```python
from build123d import *

# Parameters (mm, degrees)
BOSS_EXTRUDE1_DEPTH = 6.35
SKETCH3_R           = 2.75
CUT_EXTRUDE1_DEPTH  = 7.35


with BuildPart() as part:
    # Sketch2 → Boss-Extrude1 (new body)
    with BuildSketch(Plane(origin=(0, 0, 0), x_dir=(0, 0, -1), z_dir=(1, 0, 0))):
        Polygon((34.047619048, 160), (95.952380952, 160), (130, 50), (130, 0), (0, 0), (0, 50), align=None)
    extrude(amount=BOSS_EXTRUDE1_DEPTH)

    # Sketch3 → Cut-Extrude1 (cut, through all)
    with BuildSketch(Plane(origin=(6.35, 0, 0), x_dir=(0, 0, -1), z_dir=(1, 0, 0))):
        with Locations((10, 42.5)):
            Circle(SKETCH3_R)
        with Locations((45, 42.5)):
            Circle(SKETCH3_R)
        with Locations((10, 7.5)):
            Circle(SKETCH3_R)
        with Locations((45, 7.5)):
            Circle(SKETCH3_R)
        with Locations((120, 7.5)):
            Circle(SKETCH3_R)
        with Locations((85, 7.5)):
            Circle(SKETCH3_R)
        with Locations((85, 42.5)):
            Circle(SKETCH3_R)
        with Locations((120, 42.5)):
            Circle(SKETCH3_R)
    extrude(amount=-CUT_EXTRUDE1_DEPTH, mode=Mode.SUBTRACT)


solid = part.part
```
Model file for the job. Use its own axes, mm. Round coordinates to 2 decimals unless told otherwise and drop trailing zeros. Write each loop counter-clockwise with the first axis right and the second up, starting at its lowest first coordinate (ties: lowest second). Pieces come first, ordered by that corner, then holes. Notation, with made-up numbers: (31, 25.5) -> (40, 25.5) arc R14 cw to (40, 38.5) -> close; hole circle Ø11 at (42, 32). An arc over 180 degrees is marked (long way). Answer as CSV lines item,"result".
1. Drill centre lines: line 1 (Y direction, x = 4.5, z = -45); line 2 (Z direction, x = 1.5, y = 9); line 3 (Z direction, x = 5, y = 103). Where is each one in solid material? Low to high.
Resolved:
line 1,"0 to 4.75, 10.25 to 39.75, 45.25 to 160"
line 2,"-130 to -122.3, -117.7 to -87.3, -82.7 to -47.3, -42.7 to -12.3, -7.7 to 0"
line 3,"-113.6 to -16.4"
2. Slice it at B-B, the plane x = 3.25. State how many separate pieces and enclosed holes the cut face has, plus the area to 3 significant figures.
Resolved:
separate pieces,"1"
enclosed holes,"8"
area,"16,900 mm²"
3. Pin check, flat tips, straight feed: pin 1 Ø3 at (x, y) = (3.5, 94.5) entering from +Z; pin 2 Ø3.5 at (y, z) = (7.5, -45) entering from -X. Stop position of each tip, or through.
Resolved:
pin 1,"z = -13.31"
pin 2,"through"
4. Slice it at C-C, the plane z = -85. List the corners of the cut face in (x, y), plus the area to 3 significant figures.
Resolved:
outline,"(0, 0) -> (6.35, 0) -> (6.35, 4.75) -> (0, 4.75) -> close; (0, 10.25) -> (6.35, 10.25) -> (6.35, 39.75) -> (0, 39.75) -> close; (0, 45.25) -> (6.35, 45.25) -> (6.35, 160) -> (0, 160) -> close"
area,"946 mm²"
5. Slice it at A-A, the plane y = 42.5. List the corners of the cut face in (x, z), plus the area to 3 significant figures.
Resolved:
outline,"(0, -130) -> (6.35, -130) -> (6.35, -122.75) -> (0, -122.75) -> close; (0, -117.25) -> (6.35, -117.25) -> (6.35, -87.75) -> (0, -87.75) -> close; (0, -82.25) -> (6.35, -82.25) -> (6.35, -47.75) -> (0, -47.75) -> close; (0, -42.25) -> (6.35, -42.25) -> (6.35, -12.75) -> (0, -12.75) -> close; (0, -7.25) -> (6.35, -7.25) -> (6.35, 0) -> (0, 0) -> close"
area,"686 mm²"
6. Slice it at D-D, the plane z = -45.5. List the corners of the cut face in (x, y).
Resolved:
outline,"(0, 0) -> (6.35, 0) -> (6.35, 4.8) -> (0, 4.8) -> close; (0, 10.2) -> (6.35, 10.2) -> (6.35, 39.8) -> (0, 39.8) -> close; (0, 45.2) -> (6.35, 45.2) -> (6.35, 160) -> (0, 160) -> close"
7. Mould opens along Y. For faces 1 (the face through (6.35, 63, -66)), 2 (the face through (3.22, 6.45, -12.54)), 3 (the face through (3.131, 105.77, -112.738)) say: +Y half, -Y half, draft (parallel to the pull), parting line (faces both ways), or undercut.
Resolved:
face 1,"draft"
face 2,"undercut"
face 3,"+Y half"
